```python
from build123d import *

# Parameters (mm, degrees)
PLATE_FEATURE_DEPTH        = 5
STRAP_FEATURE_SKETCH_RX    = 18
STRAP_FEATURE_SKETCH_RY    = 8
STRAP_FEATURE_DEPTH        = 5
STRAP_CUT_SKETCH_W         = 30
STRAP_CUT_SKETCH_H         = 3.19824666
STRAP_CUT_DEPTH            = 5
LEFT_LEG_FEATURE_SKETCH_W  = 16
LEFT_LEG_FEATURE_SKETCH_H  = 8
LEFT_LEG_FEATURE_DEPTH     = 20
RIGHT_LEG_FEATURE_SKETCH_W = 16
RIGHT_LEG_FEATURE_SKETCH_H = 8
RIGHT_LEG_FEATURE_DEPTH    = 20
TAB_CUT_SKETCH_W           = 8
TAB_CUT_SKETCH_H           = 15
TAB_CUT_DEPTH              = 5
FILLET1_R                  = 10
FILLET2_R                  = 10
FILLET3_R                  = 10


with BuildPart() as part:
    # Plate Feature Sketch → Plate Feature (new body)
    with BuildSketch(Plane.XY):
        Polygon((-36, 18), (-36, 0), (-15.55368079, -50), (18.44631921, -50), (38, 0), (38, 18), align=None)
    extrude(amount=PLATE_FEATURE_DEPTH)

    # Strap Feature Sketch → Strap Feature (add)
    with BuildSketch(Plane.XY):
        with Locations((0.44631921, -50)):
            Ellipse(STRAP_FEATURE_SKETCH_RX, STRAP_FEATURE_SKETCH_RY)
    extrude(amount=STRAP_FEATURE_DEPTH)

    # Strap Cut Sketch → Strap Cut (cut)
    with BuildSketch(Plane.XY):
        with Locations((-0.034918838, -50.490814337)):
            Rectangle(STRAP_CUT_SKETCH_W, STRAP_CUT_SKETCH_H)
    extrude(amount=STRAP_CUT_DEPTH, mode=Mode.SUBTRACT)

    # Left Leg Feature Sketch → Left Leg Feature (add)
    with BuildSketch(Plane.XY):
        with Locations((30, 14)):
            Rectangle(LEFT_LEG_FEATURE_SKETCH_W, LEFT_LEG_FEATURE_SKETCH_H)
    extrude(amount=-LEFT_LEG_FEATURE_DEPTH)

    # Right Leg Feature Sketch → Right Leg Feature (add)
    with BuildSketch(Plane.XY):
        with Locations((-28, 14)):
            Rectangle(RIGHT_LEG_FEATURE_SKETCH_W, RIGHT_LEG_FEATURE_SKETCH_H)
    extrude(amount=-RIGHT_LEG_FEATURE_DEPTH)

    # Tab Cut Sketch → Tab Cut (cut)
    with BuildSketch(Plane(origin=(0, 10, 0), x_dir=(1, 0, 0), z_dir=(0, 1, 0))):
        with Locations((-28, 12.5)):
            Rectangle(TAB_CUT_SKETCH_W, TAB_CUT_SKETCH_H)
        with Locations((30, 12.5)):
            Rectangle(TAB_CUT_SKETCH_W, TAB_CUT_SKETCH_H)
    extrude(amount=TAB_CUT_DEPTH, mode=Mode.SUBTRACT)

    # Fillet1
    # the kernel refuses this fillet: 10 mm, written as the material it takes off along each edge
    with BuildSketch(Plane(origin=(63, 18, 5), x_dir=(0, 0, -1), z_dir=(-1, 0, 0))) as fillet1_piece_1:
        with BuildLine():
            CenterArc((FILLET1_R, FILLET1_R), FILLET1_R, 180, 90)
            Line((0, FILLET1_R), (0, 0))
            Line((0, 0), (FILLET1_R, 0))
        make_face()
    extrude(amount=124, mode=Mode.SUBTRACT)

    # Fillet2
    # the kernel refuses this fillet: 10 mm, written as the material it adds along each edge
    with BuildSketch(Plane(origin=(-36, 10, 0), x_dir=(0, 0, -1), z_dir=(1, 0, 0))) as fillet2_piece_1_section:
        with BuildLine():
            CenterArc((FILLET2_R, -FILLET2_R), FILLET2_R, 90, 90)
            Line((0, -FILLET2_R), (0, 0))
            Line((0, 0), (FILLET2_R, 0))
        make_face()
    fillet2_piece_1 = extrude(amount=16, mode=Mode.PRIVATE)
    fillet2_piece_1 = split(fillet2_piece_1, bisect_by=Plane(origin=(-34, 9.759916183, -5), z_dir=(0, 0, -1)), keep=Keep.TOP, mode=Mode.PRIVATE)
    fillet2_piece_1 = split(fillet2_piece_1, bisect_by=Plane(origin=(-32, 9.759916183, -6.632507845), z_dir=(-1, 0, 0)), keep=Keep.TOP, mode=Mode.PRIVATE)
    add(fillet2_piece_1)
    with BuildSketch(Plane(origin=(-36, 10, 0), x_dir=(0, 0, -1), z_dir=(1, 0, 0))) as fillet2_piece_2_section:
        with BuildLine():
            CenterArc((FILLET2_R, -FILLET2_R), FILLET2_R, 90, 90)
            Line((0, -FILLET2_R), (0, 0))
            Line((0, 0), (FILLET2_R, 0))
        make_face()
    fillet2_piece_2 = extrude(amount=16, mode=Mode.PRIVATE)
    fillet2_piece_2 = split(fillet2_piece_2, bisect_by=Plane(origin=(-34, 7.4487994, -5), z_dir=(0, 0, 1)), keep=Keep.TOP, mode=Mode.PRIVATE)
    fillet2_piece_2 = split(fillet2_piece_2, bisect_by=Plane(origin=(-32, 7.4487994, -1.643917643), z_dir=(-1, 0, 0)), keep=Keep.TOP, mode=Mode.PRIVATE)
    add(fillet2_piece_2)
    with BuildSketch(Plane(origin=(-36, 10, 0), x_dir=(0, 0, -1), z_dir=(1, 0, 0))) as fillet2_piece_3_section:
        with BuildLine():
            CenterArc((FILLET2_R, -FILLET2_R), FILLET2_R, 90, 90)
            Line((0, -FILLET2_R), (0, 0))
            Line((0, 0), (FILLET2_R, 0))
        make_face()
    fillet2_piece_3 = extrude(amount=16, mode=Mode.PRIVATE)
    fillet2_piece_3 = split(fillet2_piece_3, bisect_by=Plane(origin=(-24, 7.4487994, -1.643917643), z_dir=(-1, 0, 0)), keep=Keep.TOP, mode=Mode.PRIVATE)
    fillet2_piece_3 = split(fillet2_piece_3, bisect_by=Plane(origin=(-28, 7.4487994, -5), z_dir=(0, 0, 1)), keep=Keep.TOP, mode=Mode.PRIVATE)
    fillet2_piece_3 = split(fillet2_piece_3, bisect_by=Plane(origin=(-32, 7.4487994, -1.643917643), z_dir=(1, 0, 0)), keep=Keep.TOP, mode=Mode.PRIVATE)
    add(fillet2_piece_3)
    with BuildSketch(Plane(origin=(-36, 10, 0), x_dir=(0, 0, -1), z_dir=(1, 0, 0))) as fillet2_piece_4_section:
        with BuildLine():
            CenterArc((FILLET2_R, -FILLET2_R), FILLET2_R, 90, 90)
            Line((0, -FILLET2_R), (0, 0))
            Line((0, 0), (FILLET2_R, 0))
        make_face()
    fillet2_piece_4 = extrude(amount=16, mode=Mode.PRIVATE)
    fillet2_piece_4 = split(fillet2_piece_4, bisect_by=Plane(origin=(-24, 9.759916183, -6.632507845), z_dir=(1, 0, 0)), keep=Keep.TOP, mode=Mode.PRIVATE)
    fillet2_piece_4 = split(fillet2_piece_4, bisect_by=Plane(origin=(-22, 9.759916183, -5), z_dir=(0, 0, -1)), keep=Keep.TOP, mode=Mode.PRIVATE)
    add(fillet2_piece_4)
    with BuildSketch(Plane(origin=(-36, 10, 0), x_dir=(0, 0, -1), z_dir=(1, 0, 0))) as fillet2_piece_5_section:
        with BuildLine():
            CenterArc((FILLET2_R, -FILLET2_R), FILLET2_R, 90, 90)
            Line((0, -FILLET2_R), (0, 0))
            Line((0, 0), (FILLET2_R, 0))
        make_face()
    fillet2_piece_5 = extrude(amount=16, mode=Mode.PRIVATE)
    fillet2_piece_5 = split(fillet2_piece_5, bisect_by=Plane(origin=(-24, 7.4487994, -1.643917643), z_dir=(1, 0, 0)), keep=Keep.TOP, mode=Mode.PRIVATE)
    fillet2_piece_5 = split(fillet2_piece_5, bisect_by=Plane(origin=(-22, 7.4487994, -5), z_dir=(0, 0, 1)), keep=Keep.TOP, mode=Mode.PRIVATE)
    add(fillet2_piece_5)

    # Fillet3
    # the kernel refuses this fillet: 10 mm, written as the material it adds along each edge
    with BuildSketch(Plane(origin=(38, 10, 0), x_dir=(0, 0, -1), z_dir=(-1, 0, 0))) as fillet3_piece_1_section:
        with BuildLine():
            CenterArc((FILLET3_R, FILLET3_R), FILLET3_R, 180, 90)
            Line((0, FILLET3_R), (0, 0))
            Line((0, 0), (FILLET3_R, 0))
        make_face()
    fillet3_piece_1 = extrude(amount=16, mode=Mode.PRIVATE)
    fillet3_piece_1 = split(fillet3_piece_1, bisect_by=Plane(origin=(36, 9.759916183, -5), z_dir=(0, 0, -1)), keep=Keep.TOP, mode=Mode.PRIVATE)
    fillet3_piece_1 = split(fillet3_piece_1, bisect_by=Plane(origin=(34, 9.759916183, -6.632507845), z_dir=(1, 0, 0)), keep=Keep.TOP, mode=Mode.PRIVATE)
    add(fillet3_piece_1)
    with BuildSketch(Plane(origin=(38, 10, 0), x_dir=(0, 0, -1), z_dir=(-1, 0, 0))) as fillet3_piece_2_section:
        with BuildLine():
            CenterArc((FILLET3_R, FILLET3_R), FILLET3_R, 180, 90)
            Line((0, FILLET3_R), (0, 0))
            Line((0, 0), (FILLET3_R, 0))
        make_face()
    fillet3_piece_2 = extrude(amount=16, mode=Mode.PRIVATE)
    fillet3_piece_2 = split(fillet3_piece_2, bisect_by=Plane(origin=(36, 7.4487994, -5), z_dir=(0, 0, 1)), keep=Keep.TOP, mode=Mode.PRIVATE)
    fillet3_piece_2 = split(fillet3_piece_2, bisect_by=Plane(origin=(34, 7.4487994, -1.643917643), z_dir=(1, 0, 0)), keep=Keep.TOP, mode=Mode.PRIVATE)
    add(fillet3_piece_2)
    with BuildSketch(Plane(origin=(38, 10, 0), x_dir=(0, 0, -1), z_dir=(-1, 0, 0))) as fillet3_piece_3_section:
        with BuildLine():
            CenterArc((FILLET3_R, FILLET3_R), FILLET3_R, 180, 90)
            Line((0, FILLET3_R), (0, 0))
            Line((0, 0), (FILLET3_R, 0))
        make_face()
    fillet3_piece_3 = extrude(amount=16, mode=Mode.PRIVATE)
    fillet3_piece_3 = split(fillet3_piece_3, bisect_by=Plane(origin=(26, 7.4487994, -1.643917643), z_dir=(1, 0, 0)), keep=Keep.TOP, mode=Mode.PRIVATE)
    fillet3_piece_3 = split(fillet3_piece_3, bisect_by=Plane(origin=(30, 7.4487994, -5), z_dir=(0, 0, 1)), keep=Keep.TOP, mode=Mode.PRIVATE)
    fillet3_piece_3 = split(fillet3_piece_3, bisect_by=Plane(origin=(34, 7.4487994, -1.643917643), z_dir=(-1, 0, 0)), keep=Keep.TOP, mode=Mode.PRIVATE)
    add(fillet3_piece_3)
    with BuildSketch(Plane(origin=(38, 10, 0), x_dir=(0, 0, -1), z_dir=(-1, 0, 0))) as fillet3_piece_4_section:
        with BuildLine():
            CenterArc((FILLET3_R, FILLET3_R), FILLET3_R, 180, 90)
            Line((0, FILLET3_R), (0, 0))
            Line((0, 0), (FILLET3_R, 0))
        make_face()
    fillet3_piece_4 = extrude(amount=16, mode=Mode.PRIVATE)
    fillet3_piece_4 = split(fillet3_piece_4, bisect_by=Plane(origin=(26, 9.759916183, -6.632507845), z_dir=(-1, 0, 0)), keep=Keep.TOP, mode=Mode.PRIVATE)
    fillet3_piece_4 = split(fillet3_piece_4, bisect_by=Plane(origin=(24, 9.759916183, -5), z_dir=(0, 0, -1)), keep=Keep.TOP, mode=Mode.PRIVATE)
    add(fillet3_piece_4)
    with BuildSketch(Plane(origin=(38, 10, 0), x_dir=(0, 0, -1), z_dir=(-1, 0, 0))) as fillet3_piece_5_section:
        with BuildLine():
            CenterArc((FILLET3_R, FILLET3_R), FILLET3_R, 180, 90)
            Line((0, FILLET3_R), (0, 0))
            Line((0, 0), (FILLET3_R, 0))
        make_face()
    fillet3_piece_5 = extrude(amount=16, mode=Mode.PRIVATE)
    fillet3_piece_5 = split(fillet3_piece_5, bisect_by=Plane(origin=(26, 7.4487994, -1.643917643), z_dir=(-1, 0, 0)), keep=Keep.TOP, mode=Mode.PRIVATE)
    fillet3_piece_5 = split(fillet3_piece_5, bisect_by=Plane(origin=(24, 7.4487994, -5), z_dir=(0, 0, 1)), keep=Keep.TOP, mode=Mode.PRIVATE)
    add(fillet3_piece_5)


solid = part.part
```
Geometry: final body of the model. Coordinates: model frame, mm. A direction names the side the tool comes from. Round coordinates to 2 decimals unless told otherwise and drop trailing zeros. Order: outer loops, then holes, each group sorted by start corner. A loop starts at its lowest first (then second) coordinate and runs counter-clockwise, first axis right, second up. Notation, with made-up numbers: (-19.75, 63) -> (36.25, 63) arc R9 ccw to (36.25, 73) -> close; hole circle Ø4 at (-33, 34.5). An arc over 180 degrees is marked (long way). Write each question's results on one line, items separated by ' | '.
Q1. Ray query, line 1 along Z through (x, y) = (1, -4.5); line 2 along Y through (x, z) = (-25, -17.75); line 3 along Y through (x, z) = (-22, -12). Return the intervals inside material, ascending.
Response values:
line 1: 0 to 5 | line 2: 15 to 18 | line 3: 10 to 18
Q2. Section query D-D (y = 1.5). Output: boundary loops of the cut face in (x, z), and give its area (3 significant figures).
Response values:
outline: (-36, -0.11) -> (-20, -0.11) -> (-20, 0) -> (22, 0) -> (22, -0.11) -> (38, -0.11) -> (38, 5) -> (-36, 5) -> close | area: 374 mm²
Q3. Pull-direction query (Y, two-part tool) for faces 4 (the face through (-28, 18, -12)), 5 (the face through (0, -52.09, 2)), 6 (the face through (34, 12, -13)); classes: released by +Y, released by -Y, zero draft, split by the parting line, or undercut.
Response values:
face 4: released by +Y | face 5: undercut | face 6: zero draft
Q4. Section query A-A (z = -16.75). Output: boundary loops of the cut face in (x, y).
Response values:
outline: (-36, 10) -> (-32, 10) -> (-32, 15) -> (-24, 15) -> (-24, 10) -> (-20, 10) -> (-20, 18) -> (-36, 18) -> close; (22, 10) -> (26, 10) -> (26, 15) -> (34, 15) -> (34, 10) -> (38, 10) -> (38, 18) -> (22, 18) -> close
Q5. Section query B-B (x = 28.5). Output: boundary loops of the cut face in (y, z).
Response values:
outline: (-24.29, 0) -> (0, 0) arc R10 cw to (8.66, -5) -> (15, -5) -> (15, -20) -> (18, -20) -> (18, -5) arc R10 ccw to (8, 5) -> (-24.29, 5) -> close
Q6. Section query C-C (z = -2.5). Output: boundary loops of the cut face in (x, y), and give its area (3 significant figures).
Response values:
outline: (-36, 6.61) -> (-20, 6.61) -> (-20, 17.68) -> (-36, 17.68) -> close; (22, 6.61) -> (38, 6.61) -> (38, 17.68) -> (22, 17.68) -> close | area: 354 mm²
Q7. Pin query (flat end, axial travel): pin 1 Ø9 at (x, z) = (30.5, -12.5) entering from -Y; pin 2 Ø1 at (y, z) = (-5.5, 1.5) entering from +X; pin 3 Ø7 at (x, y) = (-29, 12.5) entering from -Z; pin 4 Ø3.5 at (y, z) = (-50.5, 3) entering from -X. Return the tip coordinate at first contact, or that it passes through.
Response values:
pin 1: y = 9.99 | pin 2: x = 36.04 | pin 3: z = -20 | pin 4: x = -17.55
Q8. Access query for faces 1 (the face through (0, -20, 0)), 2 (the face through (-22, 10, -15)), 3 (the face through (-15.035, -51, 2)). Directions: +Z, -Z, +X, -X, +Y, -Y. A direction counts if a zero-diameter tool reaches every point of the face in a straight line with its end or side. Return the directions, or none.
Response values:
face 1: -Z, -Y | face 2: -Z, +X, -X, -Y | face 3: +Z, -Z
